```python
from build123d import *

# Parameters (mm, degrees)
BOSS_EXTRUDE1_DEPTH = 34
CUT_EXTRUDE1_DEPTH  = 34
SKETCH3_W           = 19.452595801
SKETCH3_H           = 34.121613058
CUT_EXTRUDE2_DEPTH  = 67
SKETCH4_W           = 80.61958461
SKETCH4_H           = 7.775745443
CUT_EXTRUDE3_DEPTH  = 10


with BuildPart() as part:
    # Sketch1 → Boss-Extrude1 (new body)
    with BuildSketch(Plane(origin=(0, 0, 0), x_dir=(1, 0, 0), z_dir=(0, 1, 0))):
        with BuildLine():
            Line((-56, -37.75), (56, -37.75))
            ThreePointArc((56, -37.75), (58.121320344, -36.871320344), (59, -34.75))
            Line((59, -34.75), (59, 34.75))
            ThreePointArc((59, 34.75), (58.121320344, 36.871320344), (56, 37.75))
            Line((56, 37.75), (-56, 37.75))
            ThreePointArc((-56, 37.75), (-58.121320344, 36.871320344), (-59, 34.75))
            Line((-59, 34.75), (-59, -34.75))
            ThreePointArc((-59, -34.75), (-58.121320344, -36.871320344), (-56, -37.75))
        make_face()
    extrude(amount=BOSS_EXTRUDE1_DEPTH)

    # Sketch2 → Cut-Extrude1 (cut)
    with BuildSketch(Plane.XY.offset(37.75)):
        with BuildLine():
            Line((-72.082720781, 27), (-49.888346505, 27))
            ThreePointArc((-49.888346505, 27), (-47.638346505, 24.75), (-49.888346505, 22.5))
            Line((-49.888346505, 22.5), (-72.082720781, 22.5))
            ThreePointArc((-72.082720781, 22.5), (-74.332720781, 24.75), (-72.082720781, 27))
        make_face()
    cut_extrude1 = extrude(amount=-CUT_EXTRUDE1_DEPTH, mode=Mode.SUBTRACT)

    # Mirror1: Cut-Extrude1 across plane
    add(cut_extrude1.mirror(Plane(origin=(0, 0, 0), x_dir=(0, 0, 1), z_dir=(1, 0, 0))), mode=Mode.SUBTRACT)

    # Sketch3 → Cut-Extrude2 (cut)
    with BuildSketch(Plane(origin=(0, 0, -37.75), x_dir=(-1, 0, 0), z_dir=(0, 0, -1))):
        with Locations((-56.356218478, 23.676559333)):
            Rectangle(SKETCH3_W, SKETCH3_H)
    cut_extrude2 = extrude(amount=-CUT_EXTRUDE2_DEPTH, mode=Mode.SUBTRACT)

    # Mirror2: Cut-Extrude2 across plane
    add(cut_extrude2.mirror(Plane(origin=(0, 0, 0), x_dir=(0, 0, 1), z_dir=(1, 0, 0))), mode=Mode.SUBTRACT)

    # Sketch4 → Cut-Extrude3 (cut)
    with BuildSketch(Plane.XY.offset(37.75)):
        with Locations((0, 23.651152712)):
            Rectangle(SKETCH4_W, SKETCH4_H)
    extrude(amount=-CUT_EXTRUDE3_DEPTH, mode=Mode.SUBTRACT)


solid = part.part
```
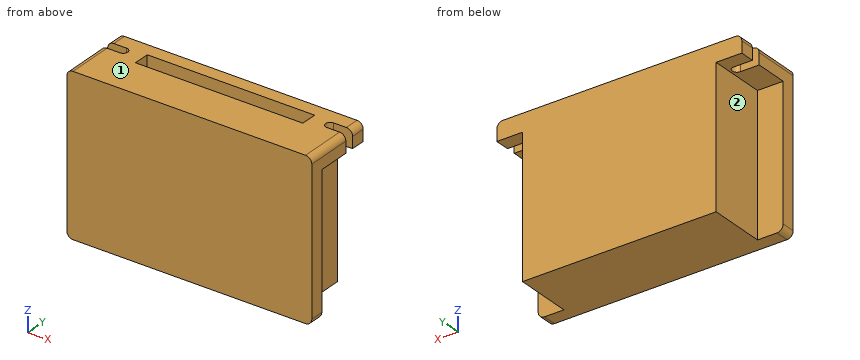
Part model, mm, in its own coordinate system. Face numbers are marked on the shaded views. A direction names the side the tool comes from. Round coordinates to 2 decimals unless told otherwise and drop trailing zeros. Write each loop counter-clockwise with the first axis right and the second up, starting at its lowest first coordinate (ties: lowest second). Pieces come first, ordered by that corner, then holes.
Item 1: Cut at B-B, the plane z = 19.5. Give the cut face in (x, y).
Results:
outline: (-59, 0) - (59, 0) - (59, 6.62) - (46.63, 6.62) - (46.63, 34) - (-46.63, 34) - (-46.63, 6.62) - (-59, 6.62) - close
Item 2: Cut at C-C, the plane y = 14. Give the cut face in (x, z), plus the area to 3 significant figures.
Results:
outline: (-59, 29.25) - (-46.63, 29.25) - (-46.63, -37.75) - (46.63, -37.75) - (46.63, 29.25) - (59, 29.25) - (59, 34.75) arc R3 ccw to (56, 37.75) - (-56, 37.75) arc R3 ccw to (-59, 34.75) - close
area: 7,250 mm2
Item 3: Probe L1, parallel to Y at x = 32.5, z = 30.5; L2, parallel to X at y = 22, z = -33.5; L3, parallel to Z at x = 23.5, y = 27. List the from-to ranges inside material, lowest first.
Results:
L1: y = 0 to 19.76, 27.54 to 34
L2: x = -46.63 to 46.63
L3: z = -37.75 to 27.75
Item 4: Which spindle directions (+Z, -Z, +X, -X, +Y, -Y) get a long thin tool onto all of the face, cutting with end or side? Do the marked faces 1 and 2. Say none if no direction does.
Results:
face 1: +Z, +X, -X, +Y, -Y
face 2: -Z, -X, +Y
Item 5: Cut at D-D, the plane x = 4.5. Give the cut face in (y, z).
Results:
outline: (0, -37.75) - (34, -37.75) - (34, 37.75) - (27.54, 37.75) - (27.54, 27.75) - (19.76, 27.75) - (19.76, 37.75) - (0, 37.75) - close
Item 6: Cut at A-A, the plane x = 51.5. Give the cut face in (y, z), plus the area to 3 significant figures.
Results:
outline: (0, -37.75) - (6.62, -37.75) - (6.62, 29.25) - (22.5, 29.25) - (22.5, 37.75) - (0, 37.75) - close; (27, 29.25) - (34, 29.25) - (34, 37.75) - (27, 37.75) - close
area: 694 mm2
Item 7: Drop flat-ended pins along their axis: pin 1 Ø6 at (x, y) = (18.5, 24) entering from +Z; pin 2 Ø6 at (x, z) = (51.5, -12.5) entering from +Y; pin 3 Ø12 at (y, z) = (30.5, 3.5) entering from -X. Give the stop position or say it passes through.
Results:
pin 1: stops at z = 27.75
pin 2: stops at y = 6.62
pin 3: stops at x = -46.63
